```python
from build123d import *

# Parameters (mm, degrees)
SKETCH008_R  = 3
PAD008_DEPTH = 6
SKETCH004_R  = 3
PAD004_DEPTH = 6
PAD001_DEPTH = 1.6
PAD_DEPTH    = 3
SKETCH002_W  = 129.8
SKETCH002_H  = 98
PAD002_DEPTH = 33
SKETCH005_R  = 3
PAD005_DEPTH = 6
SKETCH006_R  = 3
PAD006_DEPTH = 6
SKETCH007_R  = 3
PAD007_DEPTH = 6
SKETCH009_R  = 3
PAD009_DEPTH = 6
SKETCH010_R  = 3
PAD010_DEPTH = 6
SKETCH011_R  = 3
PAD011_DEPTH = 6


with BuildPart() as body008:
    # Sketch008 → Pad008 (new body)
    with BuildSketch(Plane.XY):
        with Locations((8.45, 28)):
            Circle(SKETCH008_R)
    extrude(amount=PAD008_DEPTH)


with BuildPart() as body004:
    # Sketch004 → Pad004 (new body)
    with BuildSketch(Plane.XY):
        with Locations((-53.5, 36)):
            Circle(SKETCH004_R)
    extrude(amount=PAD004_DEPTH)


with BuildPart() as body001:
    # Sketch001 → Pad001 (new body)
    with BuildSketch(Plane.XY):
        with BuildLine():
            Line((-55.5, 43.7), (61.7, 43.7))
            ThreePointArc((61.7, 43.7), (63.164466, 40.164466), (66.7, 38.7))
            Line((66.7, 38.7), (66.7, -46.7))
            ThreePointArc((66.7, -46.7), (63.164466, -48.164466), (61.7, -51.7))
            Line((61.7, -51.7), (-55.5, -51.7))
            ThreePointArc((-55.5, -51.7), (-56.964466, -48.164466), (-60.5, -46.7))
            Line((-60.5, -46.7), (-60.5, 38.7))
            ThreePointArc((-60.5, 38.7), (-56.964466, 40.164466), (-55.5, 43.7))
        make_face()
    extrude(amount=PAD001_DEPTH)


with BuildPart() as fusion:
    # Sketch → Pad (new body)
    with BuildSketch(Plane.XY):
        with BuildLine():
            Line((-61.8, 45), (-2.9, 45))
            Line((-2.9, 54), (-2.9, 45))
            ThreePointArc((9.1, 54), (3.1, 60), (-2.9, 54))
            Line((9.1, 54), (9.1, 45))
            Line((9.1, 45), (68, 45))
            Line((68, 45), (68, 2))
            Line((77, 2), (68, 2))
            ThreePointArc((77, -10), (83, -4), (77, 2))
            Line((77, -10), (68, -10))
            Line((68, -10), (68, -53))
            Line((68, -53), (9.1, -53))
            Line((9.1, -62), (9.1, -53))
            ThreePointArc((-2.9, -62), (3.1, -68), (9.1, -62))
            Line((-2.9, -62), (-2.9, -53))
            Line((-2.9, -53), (-61.8, -53))
            Line((-61.8, -53), (-61.8, -10))
            Line((-61.8, -10), (-70.8, -10))
            ThreePointArc((-70.8, 2), (-76.8, -4), (-70.8, -10))
            Line((-61.8, 2), (-70.8, 2))
            Line((-61.8, 2), (-61.8, 45))
        make_face()
        with BuildLine():
            Line((-55.5, 43.7), (61.7, 43.7))
            ThreePointArc((61.7, 43.7), (63.164466, 40.164466), (66.7, 38.7))
            Line((66.7, 38.7), (66.7, -46.7))
            ThreePointArc((66.7, -46.7), (63.164466, -48.164466), (61.7, -51.7))
            Line((61.7, -51.7), (-55.5, -51.7))
            ThreePointArc((-55.5, -51.7), (-56.964466, -48.164466), (-60.5, -46.7))
            Line((-60.5, -46.7), (-60.5, 38.7))
            ThreePointArc((-60.5, 38.7), (-56.964466, 40.164466), (-55.5, 43.7))
        make_face(mode=Mode.SUBTRACT)
    extrude(amount=PAD_DEPTH)

    # Fusion: union Body001
    add(body001.part)


with BuildPart() as fusion002:
    # Sketch002 → Pad002 (new body)
    with BuildSketch(Plane.XY):
        with Locations((3.1, -4)):
            Rectangle(SKETCH002_W, SKETCH002_H)
        with BuildLine():
            Line((-55.5, 43.7), (61.7, 43.7))
            ThreePointArc((61.7, 43.7), (63.164466, 40.164466), (66.7, 38.7))
            Line((66.7, 38.7), (66.7, -46.7))
            ThreePointArc((66.7, -46.7), (63.164466, -48.164466), (61.7, -51.7))
            Line((61.7, -51.7), (-55.5, -51.7))
            ThreePointArc((-55.5, -51.7), (-56.964466, -48.164466), (-60.5, -46.7))
            Line((-60.5, -46.7), (-60.5, 38.7))
            ThreePointArc((-60.5, 38.7), (-56.964466, 40.164466), (-55.5, 43.7))
        make_face(mode=Mode.SUBTRACT)
    extrude(amount=PAD002_DEPTH)

    # Fusion001: union Fusion
    add(fusion.part)

    # Fusion002: union Body004
    add(body004.part)


with BuildPart() as fusion003:
    # Sketch005 → Pad005 (new body)
    with BuildSketch(Plane.XY):
        with Locations((-4.5, 36)):
            Circle(SKETCH005_R)
    extrude(amount=PAD005_DEPTH)

    # Fusion003: union Fusion002
    add(fusion002.part)


with BuildPart() as fusion004:
    # Sketch006 → Pad006 (new body)
    with BuildSketch(Plane.XY):
        with Locations((-4.5, -22)):
            Circle(SKETCH006_R)
    extrude(amount=PAD006_DEPTH)

    # Fusion004: union Fusion003
    add(fusion003.part)


with BuildPart() as fusion006:
    # Sketch007 → Pad007 (new body)
    with BuildSketch(Plane.XY):
        with Locations((-53.5, -22)):
            Circle(SKETCH007_R)
    extrude(amount=PAD007_DEPTH)

    # Fusion005: union Fusion004
    add(fusion004.part)

    # Fusion006: union Body008
    add(body008.part)


with BuildPart() as fusion007:
    # Sketch009 → Pad009 (new body)
    with BuildSketch(Plane.XY):
        with Locations((56.65, 28)):
            Circle(SKETCH009_R)
    extrude(amount=PAD009_DEPTH)

    # Fusion007: union Fusion006
    add(fusion006.part)


with BuildPart() as fusion008:
    # Sketch010 → Pad010 (new body)
    with BuildSketch(Plane.XY):
        with Locations((56.65, -38)):
            Circle(SKETCH010_R)
    extrude(amount=PAD010_DEPTH)

    # Fusion008: union Fusion007
    add(fusion007.part)


with BuildPart() as fusion009:
    # Sketch011 → Pad011 (new body)
    with BuildSketch(Plane.XY):
        with Locations((8.45, -38)):
            Circle(SKETCH011_R)
    extrude(amount=PAD011_DEPTH)

    # Fusion009: union Fusion008
    add(fusion008.part)


solid = fusion009.part
```
Geometry check sheet. Reference: the model listing, model coordinates, mm. A direction names the side the tool comes from. Round coordinates to 2 decimals unless told otherwise and drop trailing zeros. Loops run counter-clockwise (first coordinate to the right, second up) from the corner with the lowest first, then second, coordinate; pieces in that order, holes last. Notation, with made-up numbers: (45.5, 22.5) - (79.5, 22.5) arc R16 ccw to (79.5, 51.5) - close; hole circle Ø1 at (32.25, -15). An arc over 180 degrees is marked (long way). Write each question's results on one line, items separated by ' | '. Start each with the question number.
Q1. Cross-section at C-C on y = -4. Enter the section's corners in (x, z).
Q2. Cross-section at D-D on y = -38. Enter the section's corners in (x, z).
Q3. Access from +Z, -Z, +X, -X, +Y, -Y to the whole of each face (thin tool, end or side, straight path). Record for faces 1 (the flat face through (-69, -4, 3)), 2 (the flat face through (57, 28, 6)), 3 (the flat face through (76, -4, 3)), 4 (the cylindrical face through (3, -68, 1)).
Q4. Cross-section at A-A on z = 26. Enter the section's corners in (x, y), and give its area (3 significant figures).
Q5. Cross-section at B-B on x = -30.5. Enter the section's corners in (y, z).
Q6. Gauge pin test, flat ends, axial feed: P1, Ø0.9, axis at y = 47.5, z = 1, coming from the +X side; P2, Ø5, axis at x = 57.5, z = 29, coming from the +Y side; P3, Ø6.5, axis at x = 8.5, y = -37.5, coming from the +Z side. Record the tip position at first contact, or that the pin passes through.
Q7. Release check for a two-part mould opening along X. For faces 5 (the cylindrical face through (-76.8, -3.9, 1.5)), 6 (the flat face through (8, 28, 6)), 7 (the cylindrical face through (-56.93, -48.2, 17.08)), 8 (the flat face through (2, 45, 16)) record: +X half, -X half, draft (parallel to the pull), parting line (faces both ways), or undercut.
Q8. Thickness scan on line 1 (X direction, y = -37.5, z = 5); line 2 (X direction, y = 27, z = 16); line 3 (Y direction, x = -24, z = 26.5). Record the ranges inside material, lowest first. Write a range as [from, to].
Answers below:
1) outline: (-76.8, 0) - (83, 0) - (83, 3) - (68, 3) - (68, 33) - (66.7, 33) - (66.7, 1.6) - (-60.5, 1.6) - (-60.5, 33) - (-61.8, 33) - (-61.8, 3) - (-76.8, 3) - close
2) outline: (-61.8, 0) - (68, 0) - (68, 33) - (66.7, 33) - (66.7, 1.6) - (59.65, 1.6) - (59.65, 6) - (53.65, 6) - (53.65, 1.6) - (11.45, 1.6) - (11.45, 6) - (5.45, 6) - (5.45, 1.6) - (-60.5, 1.6) - (-60.5, 33) - (-61.8, 33) - close
3) face 1: +Z, -X, +Y, -Y | face 2: +Z | face 3: +Z, +X, +Y, -Y | face 4: +Z, -Z, -Y
4) outline: (-61.8, -53) - (68, -53) - (68, 45) - (-61.8, 45) - close; hole (-60.5, -46.7) arc R5 cw to (-55.5, -51.7) - (61.7, -51.7) arc R5 cw to (66.7, -46.7) - (66.7, 38.7) arc R5 cw to (61.7, 43.7) - (-55.5, 43.7) arc R5 cw to (-60.5, 38.7) - close | area: 664 mm²
5) outline: (-53, 0) - (45, 0) - (45, 33) - (43.7, 33) - (43.7, 1.6) - (-51.7, 1.6) - (-51.7, 33) - (-53, 33) - close
6) P1: stops at x = 9.1 | P2: stops at y = 45 | P3: stops at z = 6
7) face 5: -X half | face 6: undercut | face 7: undercut | face 8: draft
8) line 1: x = [-61.8, -60.5], [5.49, 11.41], [53.69, 59.61], [66.7, 68] | line 2: x = [-61.8, -60.5], [66.7, 68] | line 3: y = [-53, -51.7], [43.7, 45]
